Model file for the job. Use its own axes, mm. A direction names the side the tool comes from. Coordinates: 2 decimals unless noted, no trailing zeros. Order: outer loops, then holes, each group sorted by start corner. A loop starts at its lowest first (then second) coordinate and runs counter-clockwise, first axis right, second up.
from build123d import *

# Parameters (mm, degrees)
SKETCH005_R = 1.5
PAD_DEPTH   = 3
ARRAY_COUNT = 4


with BuildPart() as revolution001:
    # Sketch004 → Revolution001 (revolve)
    with BuildSketch(Plane(origin=(0, 0, 16), x_dir=(0, 1, 0), z_dir=(1, 0, 0))):
        Polygon((20.768198, -1.5), (22.86882, 1.5), (25.36882, 1.5), (25.36882, -1.5), align=None)
    revolve(axis=Axis((0, 0, 16), (0, 0, 1)))


with BuildPart() as fusion:
    # Sketch005 → Pad (new body)
    with BuildSketch(Plane.XY.offset(14.5)):
        with BuildLine():
            ThreePointArc((20.271681, 14.630753), (17.680475, 17.674864), (14.637187, 20.267036))
            Line((14.637187, 20.267036), (16.909034, 22.538883))
            ThreePointArc((22.608377, 16.967448), (22.796148, 22.860342), (16.909034, 22.538883))
            Line((20.271681, 14.630753), (22.608377, 16.967448))
        make_face()
        with Locations((20, 20)):
            Circle(SKETCH005_R, mode=Mode.SUBTRACT)
    extrude(amount=PAD_DEPTH)

    # Array: Fusion ×4 about axis
    array_axis = Axis((0, 0, 1), (0, 0, 1))


with BuildPart() as fusion_1:
    add(fusion.part)
    for i in range(1, ARRAY_COUNT):
        add(fusion.part.rotate(array_axis, i * 360 / ARRAY_COUNT))

    # Fusion: union Revolution001
    add(revolution001.part)


solid = fusion_1.part
Q1. Probe line 1 (Y direction, x = -6.5, z = 15.3); line 2 (Y direction, x = -2.5, z = 15); line 3 (X direction, y = 16.5, z = 15.45). List the from-to ranges inside material, lowest first.
Established:
line 1: y = -24.52 to -20.31, 20.31 to 24.52
line 2: y = -25.25 to -20.97, 20.97 to 25.25
line 3: x = -22.13 to -13.68, 13.68 to 22.14
Q2. Cut at A-A, the plane y = 0. List the corners of the cut face in (x, z), plus the area to 3 significant figures.
Established:
outline: (-25.37, 14.5) - (-20.77, 14.5) - (-22.87, 17.5) - (-25.37, 17.5) - close; (20.77, 14.5) - (25.37, 14.5) - (25.37, 17.5) - (22.87, 17.5) - close
area: 21.3 mm2
Q3. Drop flat-ended pins along their axis: P1, Ø1, axis at x = 1.5, z = 15.5, coming from the +Y side; P2, Ø1.5, axis at y = 5, z = 16, coming from the +X side. Give the stop position or say it passes through.
Established:
P1: stops at y = 25.35
P2: stops at x = 25.01
Q4. Which spindle directions (+Z, -Z, +X, -X, +Y, -Y) get a long thin tool onto all of the face, cutting with end or side? Do faces 1 (the face through (15.89, 21.52, 15.98)), 2 (the face through (-21.01, 18.89, 15.98)), 3 (the face through (21.56, 15.92, 15.98)), 4 (the face through (15.92, -21.56, 15.98)), 5 (the face through (-21.52, 15.89, 15.98)). Say none if no direction does.
Established:
face 1: +Z, -Z, +Y
face 2: +Z, -Z
face 3: +Z, -Z, +X
face 4: +Z, -Z, -Y
face 5: +Z, -Z, -X
Q5. Mould opens along X. For faces 6 (the face through (18.89, 21.01, 15.98)), 7 (the face through (25.368, -0.227, 15.979)), 8 (the face through (-23, 4, 17.5)) say: pulls with the +X half, pulls with the -X half, needs draft (parallel to the pull), parting line crosses it, or undercut.
Established:
face 6: undercut
face 7: pulls with the +X half
face 8: needs draft
Q6. Cut at C-C, the plane z = 15.95. List the corners of the cut face in (x, y).
Established:
outline: (-22.61, -16.97) arc R4 ccw (long way) to (-16.91, -22.54) - (-14.9, -20.53) arc R25.37 ccw to (14.89, -20.54) - (16.97, -22.61) arc R4 ccw (long way) to (22.54, -16.91) - (20.53, -14.9) arc R25.37 ccw to (20.54, 14.89) - (22.61, 16.97) arc R4 ccw (long way) to (16.91, 22.54) - (14.9, 20.53) arc R25.37 ccw to (-14.89, 20.54) - (-16.97, 22.61) arc R4 ccw (long way) to (-22.54, 16.91) - (-20.53, 14.9) arc R25.37 ccw to (-20.54, -14.89) - close; hole circle Ø43.57 at (0, 0); hole circle Ø3 at (-20, -20); hole circle Ø3 at (-20, 20); hole circle Ø3 at (20, -20); hole circle Ø3 at (20, 20)
